from build123d import *

# Parameters (mm, degrees)
SKETCH_W        = 190
SKETCH_H        = 130
SKETCH_W_2      = 163.5
SKETCH_H_2      = 98
PAD_DEPTH       = 4
SKETCH005_W     = 190
SKETCH005_H     = 130
SKETCH005_W_2   = 186
SKETCH005_H_2   = 126
PAD002_DEPTH    = 5
POCKET_DEPTH    = 2
SKETCH006_W     = 50
SKETCH006_H     = 5
POCKET001_DEPTH = 2
FILLET_R        = 1
SKETCH010_W     = 20
SKETCH010_H     = 4
SKETCH010_W_2   = 5
PAD005_DEPTH    = 1.5


with BuildPart() as part:
    # Sketch (on DatumPlane) → Pad (new body)
    with BuildSketch(Plane.XY.offset(-2)):
        Rectangle(SKETCH_W, SKETCH_H)
        Rectangle(SKETCH_W_2, SKETCH_H_2, mode=Mode.SUBTRACT)
    extrude(amount=PAD_DEPTH)

    # Sketch005 → Pad002 (join)
    with BuildSketch(Plane.XY.offset(2)):
        Rectangle(SKETCH005_W, SKETCH005_H)
        Rectangle(SKETCH005_W_2, SKETCH005_H_2, mode=Mode.SUBTRACT)
    extrude(amount=PAD002_DEPTH)

    # Sketch003 (on Face10 of Pad) → Pocket (cut)
    with BuildSketch(Plane.XY.offset(2)):
        Polygon((-90, 52.25), (-90, -59.75), (-20, -59.75), (-20, -62.25), (20, -62.25), (20, -59.75), (86, -59.75), (86, 52.25), align=None)
    extrude(amount=-POCKET_DEPTH, mode=Mode.SUBTRACT)

    # Sketch006 (on Face2 of Pocket) → Pocket001 (cut)
    with BuildSketch(Plane(origin=(-95, 0, 0), x_dir=(0, -1, 0), z_dir=(-1, 0, 0))):
        with Locations((0, 4.5)):
            Rectangle(SKETCH006_W, SKETCH006_H)
    extrude(amount=-POCKET001_DEPTH, mode=Mode.SUBTRACT)

    # Fillet
    fillet_edges = [part.edges().sort_by_distance(p)[0] for p in [
        (0, -65, -2),
        (95, 0, -2),
        (0, 65, -2),
        (0, -49, -2),
        (81.75, 0, -2),
        (-81.75, 0, -2),
        (0, 49, -2),
        (-95, 0, -2),
        (-95, -45, 7),
        (0, -65, 7),
        (95, 0, 7),
        (0, 65, 7),
        (-95, 45, 7),
        (-94, 25, 7),
        (-94, -25, 7),
    ]]
    fillet(fillet_edges, radius=FILLET_R)

    # Sketch010 (on Face23 of Fillet) → Pad005 (join)
    with BuildSketch(Plane.XY.offset(2)):
        with Locations((-80, 53.25)):
            Rectangle(SKETCH010_W, SKETCH010_H)
        with Locations((-80, -60.75)):
            Rectangle(SKETCH010_W, SKETCH010_H)
        with Locations((86, 52.25)):
            Rectangle(SKETCH010_W_2, SKETCH010_H)
        with Locations((86, -59.75)):
            Rectangle(SKETCH010_W_2, SKETCH010_H)
    extrude(amount=PAD005_DEPTH)


solid = part.part
Source: CAD feature listing. Evaluate the final solid. Frame: model axes, mm. A direction names the side the tool comes from. Round coordinates to 2 decimals unless told otherwise and drop trailing zeros. Loops run counter-clockwise (first coordinate to the right, second up) from the corner with the lowest first, then second, coordinate; pieces in that order, holes last. Notation, with made-up numbers: M 19,-1 L 43,-1 A26 ccw 43,15 Z; hole C 49.5,48 d9. An arc over 180 degrees is marked long. Return JSON: item names as keys, results as strings. Group by question number.
1. Reachability of faces 1 (the face through (-80, 53, 3.5)), 2 (the face through (-95, -0.9, 1.7)) from +Z, -Z, +X, -X, +Y, -Y: full face, straight path, thin tool, end or side. Return the list, or none.
2. Section query B-B on y = -34. Output: boundary loops of the cut face in (x, z), and give its area (3 significant figures).
3. Material intervals for line 1 along X through (y, z) = (-58.5, 5.75); line 2 along Y through (x, z) = (-68, 5.75); line 3 along Y through (x, z) = (-82.5, 2.5), sorted ascending. Write a range as from..to.
4. Section query C-C on x = 8.5. Output: boundary loops of the cut face in (y, z).
5. Pin query (flat end, axial travel): pin 1 (2 mm diameter, centred on x = 85, y = 52, fed in from +Z); pin 2 (12 mm diameter, centred on x = -10, y = 49, fed in from +Z). Return the tip coordinate at first contact, or that it passes through.
6. Section query D-D on y = 22. Output: boundary loops of the cut face in (x, z), and give its area (3 significant figures).
7. Mould query, pull axis X, two halves, no side actions, for faces 3 (the face through (-1, 65, 2)), 4 (the face through (-93, 44, 4)), 5 (the face through (95, -1, 2)), 6 (the face through (-2, -51, 0)). Classes: released by +X, released by -X, zero draft, split by the parting line, or undercut.
Checks:
{
 "1": {"face 1": "+Z", "face 2": "+Z, -Z, -X, +Y, -Y"},
 "2": {"outline": "M -95,-1 A1 ccw -94,-2 L -82.75,-2 A1 ccw -81.75,-1 L -81.75,0 L -90,0 L -90,2 L -93,2 L -93,7 L -94,7 A1 ccw -95,6 Z; M 81.75,-1 A1 ccw 82.75,-2 L 94,-2 A1 ccw 95,-1 L 95,6 A1 ccw 94,7 L 93,7 L 93,2 L 86,2 L 86,0 L 81.75,0 Z", "area": "99.7 mm²"},
 "3": {"line 1": "x = -95..-93, 93..95", "line 2": "y = -65..-63, 63..65", "line 3": "y = -65..-63, -62.75..-58.75, 51.25..55.25, 63..65"},
 "4": {"outline": "M -65,-1 A1 ccw -64,-2 L -50,-2 A1 ccw -49,-1 L -49,0 L -62.25,0 L -62.25,2 L -63,2 L -63,7 L -64,7 A1 ccw -65,6 Z; M 49,-1 A1 ccw 50,-2 L 64,-2 A1 ccw 65,-1 L 65,6 A1 ccw 64,7 L 63,7 L 63,2 L 52.25,2 L 52.25,0 L 49,0 Z"},
 "5": {"pin 1": "stops at z = 3.5", "pin 2": "stops at z = 2"},
 "6": {"outline": "M -95,-1 A1 ccw -94,-2 L -82.75,-2 A1 ccw -81.75,-1 L -81.75,0 L -90,0 L -90,2 L -95,2 Z; M 81.75,-1 A1 ccw 82.75,-2 L 94,-2 A1 ccw 95,-1 L 95,6 A1 ccw 94,7 L 93,7 L 93,2 L 86,2 L 86,0 L 81.75,0 Z", "area": "89.9 mm²"},
 "7": {"face 3": "zero draft", "face 4": "undercut", "face 5": "released by +X", "face 6": "undercut"}
}
